Can you work these out from the model? Positions are in its coordinate system, mm. A direction names the side the tool comes from. Give positions to 0.01 mm unless a question says otherwise; leave off trailing zeros. Order: outer loops, then holes, each group sorted by start corner. A loop starts at its lowest first (then second) coordinate and runs counter-clockwise, first axis right, second up.
Item 1: If we mould it in two halves opening along Y, with no side actions, what happens to faces 3 (the flat face through (22, 19, 0)), 4 (the flat face through (-6.5, 45.22, 4.87)), 5 (the flat face through (-5, -35.62, 2))? For each: +Y half, -Y half, draft (parallel to the pull), parting line (faces both ways), or undercut.
Item 2: I want a section at C-C, the plane x = -14. Write out the boundary of the cut face in (y, z).
Item 3: I want a section at A-A, the plane y = 0. Write out the boundary of the cut face in (x, z).
Item 4: I want a section at B-B, the plane z = 6.75. Write out the boundary of the cut face in (x, y), then the cut area to 3 significant figures.
Item 5: I want a section at D-D, the plane x = -24. Write out the boundary of the cut face in (y, z), then the cut area to 3 significant figures.
Item 6: Which directions (+Z, -Z, +X, -X, +Y, -Y) give clear straight access to the entire face, cutting with the end or side of a thin tool? Please do faces 1 (the flat face through (-25.672, 0.595, 2.473)), 2 (the flat face through (22, -17, 0)).
Item 7: I'm going to push flat-ended pins straight in: pin 1 Ø3.5 at (x, z) = (-0.5, 2) entering from +Y; pin 2 Ø4 at (y, z) = (-14, 7) entering from -X; pin 3 Ø1 at (y, z) = (-26.5, 5.5) entering from -X; pin 4 Ø2 at (x, y) = (-3.5, -18.5) entering from -Z. Where does each tip first touch, or does it pass through?
Item 8: If I drill on line 1 along Y through (x, z) = (-6, 1); line 2 along Z through (x, y) = (19, -11.5); line 3 along X through (y, z) = (10, 3.25), over which ranges is the centre line in solid material (lowest first)?
```python
from build123d import *

# Parameters (mm, degrees)
F0_R          = 20.4570134616
F1_DEPTH      = 8
F3_DEPTH      = 39.9303750525
F3_DEPTH_BACK = 36.6262506595


with BuildPart() as f1:
    # F0 (on Top) → F1 (new body)
    with BuildSketch(Plane.XY):
        with BuildLine():
            Line((26.0145924985, 43.7105707824), (-39.9293750525, 46.7698224776))
            ThreePointArc((-39.9293750525, 46.7698224776), (-31.1732722705, 4.5545801964), (-39.9293750525, -37.6606620848))
            Line((-39.9293750525, -37.6606620848), (26.0145924985, -41.3985941777))
            ThreePointArc((26.0145924985, -41.3985941777), (36.6252506595, 1.1559883023), (26.0145924985, 43.7105707824))
        make_face()
        Circle(F0_R, mode=Mode.SUBTRACT)
    extrude(amount=F1_DEPTH)

    # F2 (on Right) → F3 (cut, two sides)
    with BuildSketch(Plane.YZ) as f3_sk:
        Polygon((46.8867681921, -9.8310960457), (46.8867681921, 0), (41.7443476617, 3.7811910734), (38.9640604703, 0), (33.7552301478, 3.8300217966), (30.2384872583, -0.9527491568), (23.4185017684, 4.0619454024), (19.7312268381, -0.9527491568), (13.7370294066, 3.4547483798), (11.1967735762, 0), (6.498315167, 3.4547483798), (3.9580593366, 0), (-2.8641208355, 5.0163082959), (-6.5525823368, 0), (-11.251040746, 3.4547483798), (-17.5447277725, -0.9527491568), (-20.8783004803, 3.8074266864), (-26.315116211, 0), (-28.6187960147, 3.2895400561), (-33.3160954238, 0), (-35.6197752275, 3.2895400561), (-35.6197752275, 0), (-36.6019308567, -9.8310960457), align=None)
    extrude(amount=-F3_DEPTH, mode=Mode.SUBTRACT)
    extrude(f3_sk.sketch, amount=F3_DEPTH_BACK, mode=Mode.SUBTRACT)


solid = f1.part
```
Results list:
1. face 3: draft
1. face 4: +Y half
1. face 5: undercut
2. outline: (-39.13, 0) - (-35.62, 0) - (-35.62, 3.29) - (-33.32, 0) - (-28.62, 3.29) - (-26.32, 0) - (-20.88, 3.81) - (-18.21, 0) - (-16.18, 0) - (-14.92, 0.89) - (-14.92, 8) - (-39.13, 8) - close; (14.92, 2.59) - (18.44, 0) - (20.43, 0) - (23.42, 4.06) - (28.94, 0) - (30.94, 0) - (33.76, 3.83) - (38.96, 0) - (41.74, 3.78) - (45.57, 0.97) - (45.57, 8) - (14.92, 8) - close
3. outline: (-31.27, 2.91) - (-20.46, 2.91) - (-20.46, 8) - (-31.27, 8) - close; (20.46, 2.91) - (36.62, 2.91) - (36.62, 8) - (20.46, 8) - close
4. outline: (-39.93, -37.66) - (26.01, -41.4) arc R90.64 ccw to (26.01, 43.71) - (-39.93, 46.77) arc R106.14 cw to start; hole circle Ø40.91 at (0, 0)
4. area: 4,390 mm2
5. outline: (-38.56, 0) - (-35.62, 0) - (-35.62, 3.29) - (-33.32, 0) - (-28.62, 3.29) - (-26.32, 0) - (-20.88, 3.81) - (-18.21, 0) - (-16.18, 0) - (-11.25, 3.45) - (-6.55, 0) - (-2.86, 5.02) - (3.96, 0) - (6.5, 3.45) - (11.2, 0) - (13.74, 3.45) - (18.44, 0) - (20.43, 0) - (23.42, 4.06) - (28.94, 0) - (30.94, 0) - (33.76, 3.83) - (38.96, 0) - (41.74, 3.78) - (46.03, 0.63) - (46.03, 8) - (-38.56, 8) - close
5. area: 531 mm2
6. face 1: -Z, +X, -X
6. face 2: -Z, +X, -X, +Y, -Y
7. pin 1: stops at y = 45.02
7. pin 2: stops at x = -33.18
7. pin 3: stops at x = -35.97
7. pin 4: passes through
8. line 1: y = -39.58 to -35.62, -34.02 to -31.89, -27.02 to -24.89, 19.56 to 21.17, 27.58 to 31.67, 37.6 to 39.7
8. line 2: z = 3.28 to 8
8. line 3: x = -31.31 to -17.85, 17.85 to 36.19
